from build123d import *

# Parameters (mm, degrees)
SKETCH1_R           = 1
SKETCH1_W           = 4.5
SKETCH1_H           = 4.5
SKETCH1_W_2         = 2
SKETCH1_H_2         = 5
BOSS_EXTRUDE1_DEPTH = 2.5


with BuildPart() as part:
    # Sketch1 → Boss-Extrude1 (new body, symmetric)
    with BuildSketch(Plane.XY):
        with BuildLine():
            Line((-120, -79), (-120, -20))
            ThreePointArc((-120, -20), (-117.071067812, -12.928932188), (-110, -10))
            Line((-110, -10), (-14.5, -10))
            Line((-14.5, -10), (-10, -10))
            Line((-10, -10), (-2, -10))
            Line((-2, -10), (-2, -5))
            Line((-2, -5), (-2, 0))
            Line((-2, 0), (-10, 0))
            Line((-10, 0), (-14.5, 0))
            Line((-14.5, 0), (-110, 0))
            ThreePointArc((-110, 0), (-117.071067812, 2.928932188), (-120, 10))
            Line((-120, 10), (-120, 80))
            ThreePointArc((-120, 80), (-117.071067812, 87.071067812), (-110, 90))
            Line((-110, 90), (0, 90))
            Line((0, 90), (0, 100))
            Line((0, 100), (-40, 100))
            Line((-40, 100), (-44.5, 100))
            Line((-44.5, 100), (-120, 100))
            Line((-120, 100), (-130, 100))
            ThreePointArc((-130, 100), (-137.071067812, 97.071067812), (-140, 90))
            Line((-140, 90), (-140, -195))
            ThreePointArc((-140, -195), (-138.535533906, -198.535533906), (-135, -200))
            Line((-135, -200), (-125, -200))
            ThreePointArc((-125, -200), (-121.464466094, -198.535533906), (-120, -195))
            Line((-120, -195), (-120, -120))
            Line((-120, -120), (-120, -110))
            Line((-120, -110), (-120, -100))
            Line((-120, -100), (-132, -100))
            Line((-132, -100), (-132, -79))
            Line((-132, -79), (-120, -79))
        make_face()
        with Locations((-126, -102)):
            Circle(SKETCH1_R, mode=Mode.SUBTRACT)
        with Locations((-126, -77)):
            Circle(SKETCH1_R, mode=Mode.SUBTRACT)
        with Locations((-42.25, 102.25)):
            Rectangle(SKETCH1_W, SKETCH1_H)
        with Locations((-12.25, 2.25)):
            Rectangle(SKETCH1_W, SKETCH1_H)
        with Locations((-12.25, -12.25)):
            Rectangle(SKETCH1_W, SKETCH1_H)
        with Locations((-1, -2.5)):
            Rectangle(SKETCH1_W_2, SKETCH1_H_2)
        Polygon((-14.5, -110), (-120, -110), (-120, -120), (-2.5, -120), (-2.5, -110), (-10, -110), align=None)
        with Locations((-12.25, -107.75)):
            Rectangle(SKETCH1_W, SKETCH1_H)
    extrude(amount=BOSS_EXTRUDE1_DEPTH, both=True)

    # Mirror1: part across plane


with BuildPart() as part_1:
    add(part.part)
    add(part.part.mirror(Plane(origin=(0, 0, 0), x_dir=(0, 0, 1), z_dir=(1, 0, 0))))


solid = part_1.part
Geometry: final body of the model. Coordinates: model frame, mm. A direction names the side the tool comes from. Give positions to 0.01 mm unless a question says otherwise; leave off trailing zeros. Write each loop counter-clockwise with the first axis right and the second up, starting at its lowest first coordinate (ties: lowest second). Pieces come first, ordered by that corner, then holes.
(1) Access query for faces 4 (the cylindrical face through (-117.15, 86.99, 0.04)), 5 (the flat face through (11, -13, -2.5)). Directions: +Z, -Z, +X, -X, +Y, -Y. A direction counts if a zero-diameter tool reaches every point of the face in a straight line with its end or side. Return the directions, or none.
(2) Cut plane B-B, the plane z = 0.75. Give the number of separate pieces and of enclosed holes in the cut face, then the cut area to 3 significant figures.
(3) First-contact query: P1, Ø1.3, axis at x = 12, z = 1, coming from the -Y side; P2, Ø1.3, axis at y = 103, z = -1, coming from the +X side. Flat tips, straight axial feed; report the tip coordinate or a pass-through.
(4) Mould query, pull axis X, two halves, no side actions, for faces 1 (the flat face through (11, -13, 2.5)), 2 (the cylindrical face through (-136.99, 97.15, 0.04)), 3 (the cylindrical face through (-117.15, -13.01, 0.04)). Classes: released by +X, released by -X, zero draft, split by the parting line, or undercut.
(5) Ray query, line 1 (Y direction, x = 126, z = 1.3); line 2 (X direction, y = -77, z = 1.35); line 3 (Y direction, x = 33.5, z = -1.9). Return the intervals inside material, ascending.
(6) Cut plane A-A, the plane y = -85. Return loops of the section in (x, z), then the cut area to 3 significant figures.
(7) Cut plane C-C, the plane y = -175. Return loops of the section in (x, z).
Values follow:
1. face 4: +Z, -Z
1. face 5: -Z, +X, -X, +Y, -Y
2. separate pieces: 1
2. enclosed holes: 5
2. area: 18,800 mm2
3. P1: stops at y = -120
3. P2: stops at x = 44.5
4. face 1: zero draft
4. face 2: released by -X
4. face 3: undercut
5. line 1: y = -200 to -103, -101 to -100, -79 to -78, -76 to 100
5. line 2: x = -140 to -127, -125 to -120, 120 to 125, 127 to 140
5. line 3: y = -120 to -110, -10 to 0, 90 to 100
6. outline: (-140, -2.5) - (-132, -2.5) - (-132, 2.5) - (-140, 2.5) - close; (132, -2.5) - (140, -2.5) - (140, 2.5) - (132, 2.5) - close
6. area: 80.0 mm2
7. outline: (-140, -2.5) - (-120, -2.5) - (-120, 2.5) - (-140, 2.5) - close; (120, -2.5) - (140, -2.5) - (140, 2.5) - (120, 2.5) - close
